from build123d import *

# Parameters (mm, degrees)
BOSS_EXTRUDE1_DEPTH                            = 38.1
CBORE_FOR_8_SOCKET_HEAD_CAP_SCREW1_D           = 4.4958
CBORE_FOR_8_SOCKET_HEAD_CAP_SCREW1_CBORE_D     = 7.9375
CBORE_FOR_8_SOCKET_HEAD_CAP_SCREW1_CBORE_DEPTH = 4.1656
CUT_EXTRUDE1_DEPTH                             = 59.695987222
F_6_CLEARANCE_HOLE1_D                          = 3.7973
CUT_EXTRUDE2_DEPTH                             = 59.695987222
SKETCH6_W                                      = 9.906
SKETCH6_H                                      = 12.7
CUT_EXTRUDE3_DEPTH                             = 3.81


with BuildPart() as part:
    # Sketch1 → Boss-Extrude1 (new body)
    with BuildSketch(Plane(origin=(0, 0, 0), x_dir=(1, 0, 0), z_dir=(0, 1, 0))):
        Polygon((0, 0), (6.35, 0), (6.35, -3.81), (44.196, -3.81), (44.196, -0.814646677), (44.196, 2.54), (0, 2.54), align=None)
    extrude(amount=BOSS_EXTRUDE1_DEPTH)

    # CBORE for #8 Socket Head Cap Screw1 (through all)
    with Locations(Plane(origin=(37.846, 31.75, -2.54), x_dir=(-1, 0, 0), z_dir=(0, 0, -1))):
        with Locations((0, 0), (0, -25.4)):
            CounterBoreHole(CBORE_FOR_8_SOCKET_HEAD_CAP_SCREW1_D / 2, CBORE_FOR_8_SOCKET_HEAD_CAP_SCREW1_CBORE_D / 2, CBORE_FOR_8_SOCKET_HEAD_CAP_SCREW1_CBORE_DEPTH)

    # Sketch3 → Cut-Extrude1 (cut, through all)
    with BuildSketch(Plane(origin=(0, 0, -2.54), x_dir=(-1, 0, 0), z_dir=(0, 0, -1))):
        Polygon((0, 29.21), (-18.796, 38.1), (0, 38.1), align=None)
        Polygon((0, 8.89), (-18.796, 0), (0, 0), align=None)
    extrude(amount=-CUT_EXTRUDE1_DEPTH, mode=Mode.SUBTRACT)

    # #6 Clearance Hole1 (through all)
    with Locations(Plane(origin=(2.921, 26.035, -2.54), x_dir=(-1, 0, 0), z_dir=(0, 0, -1))):
        with Locations((0, 0), (0, -13.97)):
            Hole(F_6_CLEARANCE_HOLE1_D / 2)

    # Sketch5 → Cut-Extrude2 (cut, through all)
    with BuildSketch(Plane(origin=(0, 0, -2.54), x_dir=(-1, 0, 0), z_dir=(0, 0, -1))):
        with BuildLine():
            Line((-16.256, 12.7), (-44.196, 12.7))
            Line((-44.196, 12.7), (-44.196, 25.4))
            Line((-44.196, 25.4), (-16.256, 25.4))
            ThreePointArc((-16.256, 25.4), (-9.906, 19.05), (-16.256, 12.7))
        make_face()
    extrude(amount=-CUT_EXTRUDE2_DEPTH, mode=Mode.SUBTRACT)

    # Sketch6 → Cut-Extrude3 (cut)
    with BuildSketch(Plane.XY.offset(3.81)):
        with Locations((11.303, 19.05)):
            Rectangle(SKETCH6_W, SKETCH6_H)
    extrude(amount=-CUT_EXTRUDE3_DEPTH, mode=Mode.SUBTRACT)


solid = part.part
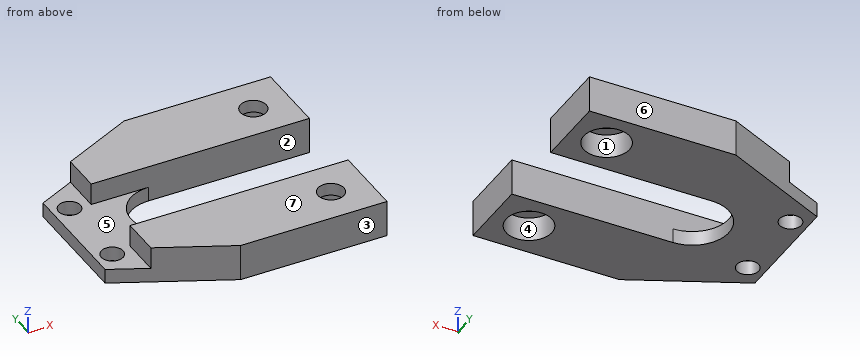
Read the model definition and answer for the solid it produces. Units are mm, in the model's axes. Face numbers are marked on the shaded views. A direction names the side the tool comes from. Round coordinates to 2 decimals unless told otherwise and drop trailing zeros. Order: outer loops, then holes, each group sorted by start corner. A loop starts at its lowest first (then second) coordinate and runs counter-clockwise, first axis right, second up.
1) The part is cut by section B-B on x = 31.5. Write down the section's boundary in (y, z), plus the area to 3 significant figures.
2) The part is cut by section C-C on y = 30. Write down the section's boundary in (x, z), plus the area to 3 significant figures.
3) For the marked faces 1, 2 and 3, determine the directions among +Z, -Z, +X, -X, +Y, -Y from which every point of the face is accessible in a straight line to the end or side of a thin tool.
4) Straight lines are drawn through the part: L1, parallel to Y at x = 42.5, z = 0.5; L2, parallel to Y at x = 38.5, z = 3.25; L3, parallel to X at y = 32, z = 1.5. For each, find the intervals that lie inside material, in ascending order.
5) Flat-ended cylindrical pins translate along their axes: pin 1 (1 mm diameter, centred on y = 32, z = 1.5, fed in from -X); pin 2 (4 mm diameter, centred on x = 38, y = 5.5, fed in from -Z). Find the tip coordinate at first contact, or state that the pin passes through.
6) The part is cut by section D-D on y = 11.5. Write down the section's boundary in (x, z), plus the area to 3 significant figures.
7) The mould has two halves that part along Y. Classify the marked faces 4, 5, 6 and 7: released by +Y, released by -Y, zero draft, split by the parting line, or undercut.
8) The part is cut by section A-A on z = 2.25. Write down the section's boundary in (x, y), plus the area to 3 significant figures.
Resolved:
1. outline: (0, -2.54) - (12.7, -2.54) - (12.7, 3.81) - (0, 3.81) - close; (25.4, -2.54) - (38.1, -2.54) - (38.1, 3.81) - (25.4, 3.81) - close
1. area: 161 mm2
2. outline: (1.67, -2.54) - (34.28, -2.54) - (34.28, 1.63) - (36.44, 1.63) - (36.44, 3.81) - (6.35, 3.81) - (6.35, 0) - (1.67, 0) - close; (39.26, 1.63) - (41.41, 1.63) - (41.41, -2.54) - (44.2, -2.54) - (44.2, 3.81) - (39.26, 3.81) - close
2. area: 216 mm2
3. face 1: -Z
3. face 2: +Z, +X
3. face 3: +Z, -Z, +X, -X, -Y
4. L1: y = 0 to 12.7, 25.4 to 38.1
4. L2: y = 0 to 4.2, 8.5 to 12.7, 25.4 to 29.6, 33.9 to 38.1
4. L3: x = 6.35 to 33.89, 41.81 to 44.2
5. pin 1: stops at x = 6.35
5. pin 2: stops at z = 1.63
6. outline: (0, -2.54) - (1.11, -2.54) - (1.11, 0) - (0, 0) - close; (4.73, -2.54) - (44.2, -2.54) - (44.2, 3.81) - (6.35, 3.81) - (6.35, 0) - (4.73, 0) - close
6. area: 247 mm2
7. face 4: undercut
7. face 5: undercut
7. face 6: released by +Y
7. face 7: zero draft
8. outline: (6.35, 5.89) - (18.8, 0) - (44.2, 0) - (44.2, 12.7) - (6.35, 12.7) - close; (6.35, 25.4) - (44.2, 25.4) - (44.2, 38.1) - (18.8, 38.1) - (6.35, 32.21) - close; hole circle Ø4.5 at (37.85, 6.35); hole circle Ø4.5 at (37.85, 31.75)
8. area: 856 mm2
